Here's how the part is built. I have some questions about the finished solid (model axes, mm). A direction names the side the tool comes from. Give positions to 0.01 mm unless a question says otherwise; leave off trailing zeros. Write each loop counter-clockwise with the first axis right and the second up, starting at its lowest first coordinate (ties: lowest second). Pieces come first, ordered by that corner, then holes. Notation, with made-up numbers: (-34, 22) - (-12, 22) arc R31 ccw to (-12, 54) - close; hole circle Ø1 at (-31, -5). An arc over 180 degrees is marked (long way). Write each question's results on one line, items separated by ' | '. Start each with the question number.
Item 1: Suppose I cut it at C-C on y = 4.25. List the corners of the cut face in (x, z) for me, then the cut area to 3 significant figures.
Item 2: Which directions (+Z, -Z, +X, -X, +Y, -Y) give clear straight access to the entire face, cutting with the end or side of a thin tool? Please do faces 1 (the flat face through (-15.508, 1, 8)), 2 (the flat face through (-28, 0, 10)), 3 (the flat face through (34.592, 6, 8)).
Item 3: Please list where these lines run through material, in increasing order: line 1 along X through (y, z) = (-1.25, 8); line 2 along X through (y, z) = (4.5, 12.75); line 3 along X through (y, z) = (-1.5, 2.5).
Item 4: Suppose I cut it at D-D on z = 2.5. List the corners of the cut face in (x, y) for me.
Item 5: Suppose I cut it at A-A on y = -2.5. List the corners of the cut face in (x, z) for me.
Item 6: Will these pins go through, and if not, where does the flat tip stop? P1, Ø8, axis at x = 2.5, z = 5, coming from the -Y side; P2, Ø5, axis at x = 45, z = 4, coming from the +Y side; P3, Ø4, axis at y = 6.5, z = 8, coming from the -X side.
Item 7: We'd pull the mould along Z, two halves only. Please class faces 4 (the flat face through (50.592, -2, 8)), 5 (the flat face through (7, 9, 0)), 6 (the cylindrical face through (-29.35, -2.16, 7.61)): +Z half, -Z half, draft (parallel to the pull), parting line (faces both ways), or undercut.
Item 8: Suppose I cut it at B-B on z = 8. List the corners of the cut face in (x, y) for me.
```python
from build123d import *

# Parameters (mm, degrees)
EXTRUDE_1_DEPTH = 16
SKETCH_3_W      = 16
SKETCH_3_H      = 4.26667426
EXTRUDE_3_DEPTH = 16
SKETCH_23_W     = 16
SKETCH_23_H     = 4.26667426
EXTRUDE_4_DEPTH = 16
F_2_0MM_2_D     = 2.6
F_2_0MM_3_D     = 2.6
SKETCH_33_W     = 45.5
SKETCH_33_H     = 16
EXTRUDE_5_DEPTH = 1


with BuildPart() as part:
    # 草图2 → 凸台-拉伸1 (new body)
    with BuildSketch(Plane.XY):
        Polygon((34.591799544, 12.66332574), (-20.108200456, 12.66332574), (-20.108200456, -4.26667426), (-15.508200456, -4.26667426), (-15.508200456, 8.06332574), (29.991799544, 8.06332574), (29.991799544, -4.26667426), (34.591799544, -4.26667426), align=None)
    extrude(amount=EXTRUDE_1_DEPTH)

    # 草图3 → 凸台-拉伸3 (add)
    with BuildSketch(Plane.ZY.offset(20.108200456)):
        with Locations((8, -2.13333713)):
            Rectangle(SKETCH_3_W, SKETCH_3_H)
    extrude(amount=EXTRUDE_3_DEPTH)

    # 草图23 → 凸台-拉伸4 (add)
    with BuildSketch(Plane(origin=(34.591799544, 0, 0), x_dir=(0, 0, -1), z_dir=(1, 0, 0))):
        with Locations((-8, -2.13333713)):
            Rectangle(SKETCH_23_W, SKETCH_23_H)
    extrude(amount=EXTRUDE_4_DEPTH)

    # Ø2.0mm 暗销孔2 (through all)
    with Locations(Plane(origin=(0, 0, 0), x_dir=(1, 0, 0), z_dir=(0, 1, 0))):
        with Locations((42.591799544, -8)):
            Hole(F_2_0MM_2_D / 2)

    # Ø2.0mm 暗销孔3 (through all)
    with Locations(Plane(origin=(0, 0, 0), x_dir=(1, 0, 0), z_dir=(0, 1, 0))):
        with Locations((-28.108200456, -8)):
            Hole(F_2_0MM_3_D / 2)

    # 草图33 → 凸台-拉伸5 (add)
    with BuildSketch(Plane.XZ.offset(-8.06332574)):
        with Locations((7.241799544, 8)):
            Rectangle(SKETCH_33_W, SKETCH_33_H)
    extrude(amount=EXTRUDE_5_DEPTH)


solid = part.part
```
Checked values:
1) outline: (-20.11, 0) - (-15.51, 0) - (-15.51, 16) - (-20.11, 16) - close; (29.99, 0) - (34.59, 0) - (34.59, 16) - (29.99, 16) - close | area: 147 mm^2
2) face 1: +Z, -Z, -Y | face 2: +Z, -Z, -X, +Y | face 3: +Z, -Z, +X, +Y
3) line 1: x = -36.11 to -29.41, -26.81 to -15.51, 29.99 to 41.29, 43.89 to 50.59 | line 2: x = -20.11 to -15.51, 29.99 to 34.59 | line 3: x = -36.11 to -15.51, 29.99 to 50.59
4) outline: (-36.11, -4.27) - (-15.51, -4.27) - (-15.51, 7.06) - (29.99, 7.06) - (29.99, -4.27) - (50.59, -4.27) - (50.59, 0) - (34.59, 0) - (34.59, 12.66) - (-20.11, 12.66) - (-20.11, 0) - (-36.11, 0) - close
5) outline: (-36.11, 0) - (-15.51, 0) - (-15.51, 16) - (-36.11, 16) - close; (29.99, 0) - (50.59, 0) - (50.59, 16) - (29.99, 16) - close; hole circle Ø2.6 at (-28.11, 8); hole circle Ø2.6 at (42.59, 8)
6) P1: stops at y = 7.06 | P2: stops at y = 0 | P3: stops at x = -20.11
7) face 4: draft | face 5: -Z half | face 6: undercut
8) outline: (-36.11, -4.27) - (-29.41, -4.27) - (-29.41, 0) - (-36.11, 0) - close; (-26.81, -4.27) - (-15.51, -4.27) - (-15.51, 7.06) - (29.99, 7.06) - (29.99, -4.27) - (41.29, -4.27) - (41.29, 0) - (34.59, 0) - (34.59, 12.66) - (-20.11, 12.66) - (-20.11, 0) - (-26.81, 0) - close; (43.89, -4.27) - (50.59, -4.27) - (50.59, 0) - (43.89, 0) - close
